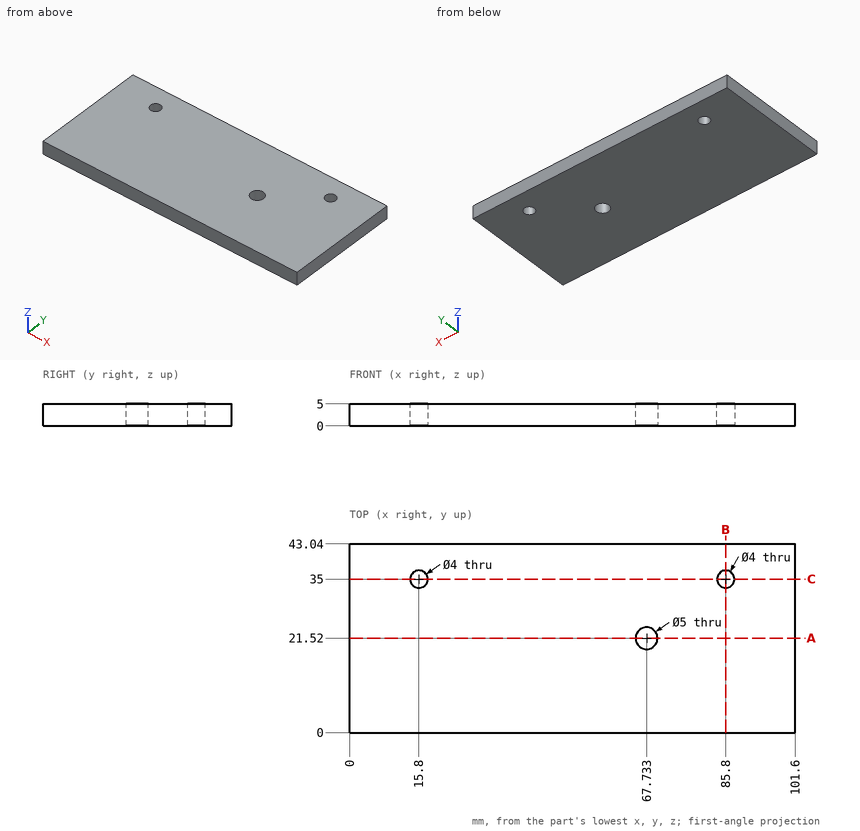
For this review, use the dimensioned drawing (mm, ordinates from the lowest corner) and the shaded views. Coordinates: 2 decimals unless noted, no trailing zeros. Loops run counter-clockwise (first coordinate to the right, second up) from the corner with the lowest first, then second, coordinate; pieces in that order, holes last. Notation, with made-up numbers: (-14.75, 0.5) -> (11.25, 0.5) arc R35 ccw to (11.25, 32.5) -> close; hole circle Ø9 at (-2, 79). An arc over 180 degrees is marked (long way). Return JSON: item names as keys, results as strings. Group by question number.
(1) Consider section B-B, the plane x = 85.8. Give the boundary of the cut face in (y, z), plus the area to 3 significant figures.
(2) To check wall thickness, follow L1, parallel to Y at x = 86, z = 1.9; L2, parallel to Y at x = 67.5, z = 4.7. State the ranges of each line that lie inside material, in increasing order.
(3) Consider section A-A, the plane y = 21.52. Give the boundary of the cut face in (x, z), plus the area to 3 significant figures.
(4) Consider section C-C, the plane y = 35. Give the boundary of the cut face in (x, z).
(5) For pin 1 Ø4 at (x, y) = (67.73, 21.52) entering from +Z; pin 2 Ø5 at (x, y) = (40, 18.5) entering from -Z, all flat-tipped, find the tip position at first contact; note any pin that passes through.
Results below:
{
 "1": {"outline": "(0, 0) -> (33, 0) -> (33, 5) -> (0, 5) -> close; (37, 0) -> (43.04, 0) -> (43.04, 5) -> (37, 5) -> close", "area": "195 mm2"},
 "2": {"L1": "y = 0 to 33.01, 36.99 to 43.04", "L2": "y = 0 to 19.03, 24.01 to 43.04"},
 "3": {"outline": "(0, 0) -> (65.23, 0) -> (65.23, 5) -> (0, 5) -> close; (70.23, 0) -> (101.6, 0) -> (101.6, 5) -> (70.23, 5) -> close", "area": "483 mm2"},
 "4": {"outline": "(0, 0) -> (13.8, 0) -> (13.8, 5) -> (0, 5) -> close; (17.8, 0) -> (83.8, 0) -> (83.8, 5) -> (17.8, 5) -> close; (87.8, 0) -> (101.6, 0) -> (101.6, 5) -> (87.8, 5) -> close"},
 "5": {"pin 1": "passes through", "pin 2": "stops at z = 0"}
}
